Read the model definition and answer for the solid it produces. Units are mm, in the model's axes. Face numbers are marked on the shaded views. A direction names the side the tool comes from. Round coordinates to 2 decimals unless told otherwise and drop trailing zeros. Order: outer loops, then holes, each group sorted by start corner. A loop starts at its lowest first (then second) coordinate and runs counter-clockwise, first axis right, second up. Notation, with made-up numbers: (37, 44.5) - (46, 44.5) arc R21 ccw to (46, 83.5) - close; hole circle Ø4 at (-23.75, 34.25). An arc over 180 degrees is marked (long way). Answer as a JSON object with one key per item and string values. Group by question number.
Q1. A cutting plane is placed at D-D on x = 13. Determine the outline of the cut face in (y, z).
Q2. Consider line 1 (Z direction, x = 43, y = 2.5); line 2 (Z direction, x = 31.5, y = 14); line 3 (X direction, y = 8, z = 31.5). Determine where each line is inside the solid, lowest interval first.
Q3. A cutting plane is placed at A-A on z = 21. Determine the outline of the cut face in (x, y), and give its area (3 significant figures).
Q4. A cutting plane is placed at C-C on y = 16. Determine the outline of the cut face in (x, z).
Q5. The mould has two halves that part along X. Classify the marked faces 4, 5, 6 and 7: pulls with the +X half, pulls with the -X half, needs draft (parallel to the pull), parting line crosses it, or undercut.
Q6. Given pin 1 Ø2 at (y, z) = (5, 14) entering from -X; pin 2 Ø1.4 at (y, z) = (12.5, 40) entering from +X, each flat-ended and moving along its own axis, determine where each tip first touches the part or whether it passes through.
Q7. A tool of negligible diameter and unlimited length cuts with its end or side. For the marked faces 1, 2 and 3, from which of +Z, -Z, +X, -X, +Y, -Y can it reach the whole face along a straight path? Write none if from no direction.
Q8. A cutting plane is placed at B-B on x = 46. Determine the outline of the cut face in (y, z).
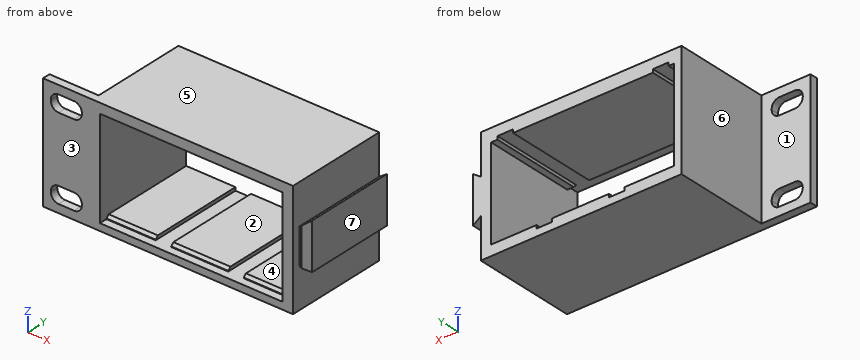
```python
from build123d import *

# Parameters (mm, degrees)
BOX027_W               = 71
BOX027_H               = 10
BOX027_DEPTH           = 10
BOX027_PLACEMENT_ANGLE = 45
BOX022_W               = 22
BOX022_H               = 37
BOX022_DEPTH           = 4
BOX023_W               = 18
BOX023_H               = 37
BOX023_DEPTH           = 4
BOX021_W               = 19
BOX021_H               = 37
BOX021_DEPTH           = 4
BOX028_W               = 80
BOX028_H               = 10
BOX028_DEPTH           = 10
BOX028_PLACEMENT_ANGLE = 315
BOX025_W               = 3
BOX025_H               = 37
BOX025_DEPTH           = 4
BOX026_W               = 4
BOX026_H               = 37
BOX026_DEPTH           = 4
BOX024_W               = 54
BOX024_H               = 37
BOX024_DEPTH           = 4
BOX019_W               = 12
BOX019_H               = 10
BOX019_DEPTH           = 6.3
FILLET_R               = 3
BOX020_W               = 12
BOX020_H               = 10
BOX020_DEPTH           = 6.3
FILLET001_R            = 3
BOX018_W               = 19
BOX018_H               = 37
BOX018_DEPTH           = 45
BOX017_W               = 70.5
BOX017_H               = 45
BOX017_DEPTH           = 37.95
BOX016_W               = 96.5
BOX016_H               = 40
BOX016_DEPTH           = 44.5
BOX013_W               = 3
BOX013_H               = 37
BOX013_DEPTH           = 17.92
BOX013_PLACEMENT_ANGLE = 45
BOX014_W               = 3
BOX014_H               = 37
BOX014_DEPTH           = 17.92
BOX014_PLACEMENT_ANGLE = 55
BOX015_W               = 3
BOX015_H               = 37
BOX015_DEPTH           = 17.92
BOX015_PLACEMENT_ANGLE = 125
BOX012_W               = 3
BOX012_H               = 37
BOX012_DEPTH           = 17.92
CUT007_PLACEMENT_ANGLE = 180


with BuildPart() as cube027:
    # Box027 → Box027 (new body)
    with BuildSketch(Plane.XY):
        with Locations((35.5, 5)):
            Rectangle(BOX027_W, BOX027_H)
    extrude(amount=BOX027_DEPTH)


with BuildPart() as cube027_1:
    # Box027 placement: moved
    add(cube027.part.moved(Location((22, -3, 0))).rotate(Axis((22, -3, 0), (1, 0, 0)), BOX027_PLACEMENT_ANGLE))


with BuildPart() as cube022:
    # Box022 → Box022 (new body)
    with BuildSketch(Plane(origin=(47, 0, 0), x_dir=(1, 0, 0), z_dir=(0, 0, 1))):
        with Locations((11, 18.5)):
            Rectangle(BOX022_W, BOX022_H)
    extrude(amount=BOX022_DEPTH)


with BuildPart() as cube023:
    # Box023 → Box023 (new body)
    with BuildSketch(Plane(origin=(75, 0, 0), x_dir=(1, 0, 0), z_dir=(0, 0, 1))):
        with Locations((9, 18.5)):
            Rectangle(BOX023_W, BOX023_H)
    extrude(amount=BOX023_DEPTH)


with BuildPart() as cut010:
    # Box021 → Box021 (new body)
    with BuildSketch(Plane(origin=(22, 0, 0), x_dir=(1, 0, 0), z_dir=(0, 0, 1))):
        with Locations((9.5, 18.5)):
            Rectangle(BOX021_W, BOX021_H)
    extrude(amount=BOX021_DEPTH)

    # Fusion005: union Cube022, Cube023
    add(cube022.part)
    add(cube023.part)

    # Cut010: cut Cube027
    add(cube027_1.part, mode=Mode.SUBTRACT)


with BuildPart() as cube028:
    # Box028 → Box028 (new body)
    with BuildSketch(Plane.XY):
        with Locations((40, 5)):
            Rectangle(BOX028_W, BOX028_H)
    extrude(amount=BOX028_DEPTH)


with BuildPart() as cube028_1:
    # Box028 placement: moved
    add(cube028.part.moved(Location((13, -8, 35))).rotate(Axis((13, -8, 35), (1, 0, 0)), BOX028_PLACEMENT_ANGLE))


with BuildPart() as cube025:
    # Box025 → Box025 (new body)
    with BuildSketch(Plane(origin=(21.05, 0, 39.45), x_dir=(1, 0, 0), z_dir=(0, 0, 1))):
        with Locations((1.5, 18.5)):
            Rectangle(BOX025_W, BOX025_H)
    extrude(amount=BOX025_DEPTH)


with BuildPart() as cube026:
    # Box026 → Box026 (new body)
    with BuildSketch(Plane(origin=(90.05, 0, 39.45), x_dir=(1, 0, 0), z_dir=(0, 0, 1))):
        with Locations((2, 18.5)):
            Rectangle(BOX026_W, BOX026_H)
    extrude(amount=BOX026_DEPTH)


with BuildPart() as cut011:
    # Box024 → Box024 (new body)
    with BuildSketch(Plane(origin=(30.05, 0, 39.45), x_dir=(1, 0, 0), z_dir=(0, 0, 1))):
        with Locations((27, 18.5)):
            Rectangle(BOX024_W, BOX024_H)
    extrude(amount=BOX024_DEPTH)

    # Fusion006: union Cube025, Cube026
    add(cube025.part)
    add(cube026.part)

    # Cut011: cut Cube028
    add(cube028_1.part, mode=Mode.SUBTRACT)


with BuildPart() as fillet_body:
    # Box019 → Box019 (new body)
    with BuildSketch(Plane(origin=(3, -3, 3.2), x_dir=(1, 0, 0), z_dir=(0, 0, 1))):
        with Locations((6, 5)):
            Rectangle(BOX019_W, BOX019_H)
    extrude(amount=BOX019_DEPTH)

    # Fillet
    fillet_edges = [fillet_body.edges().sort_by_distance(p)[0] for p in [
        (3, 2, 9.5),
        (3, 2, 3.2),
        (15, 2, 9.5),
        (15, 2, 3.2),
    ]]
    fillet(fillet_edges, radius=FILLET_R)


with BuildPart() as fillet_body_1:
    # Fillet placement: moved
    add(fillet_body.part.moved(Location((0, -1, 0))))


with BuildPart() as fillet001:
    # Box020 → Box020 (new body)
    with BuildSketch(Plane(origin=(3, -3, 3.2), x_dir=(1, 0, 0), z_dir=(0, 0, 1))):
        with Locations((6, 5)):
            Rectangle(BOX020_W, BOX020_H)
    extrude(amount=BOX020_DEPTH)

    # Fillet001
    fillet001_edges = [fillet001.edges().sort_by_distance(p)[0] for p in [
        (3, 2, 9.5),
        (3, 2, 3.2),
        (15, 2, 9.5),
        (15, 2, 3.2),
    ]]
    fillet(fillet001_edges, radius=FILLET001_R)


with BuildPart() as fillet001_1:
    # Fillet001 placement: moved
    add(fillet001.part.moved(Location((0, -1, 31.7))))


with BuildPart() as fusion004:
    # Box018 → Box018 (new body)
    with BuildSketch(Plane.XY):
        with Locations((9.5, 18.5)):
            Rectangle(BOX018_W, BOX018_H)
    extrude(amount=BOX018_DEPTH)

    # Fusion004: union Fillet body, Fillet001
    add(fillet_body_1.part)
    add(fillet001_1.part)


with BuildPart() as cube017:
    # Box017 → Box017 (new body)
    with BuildSketch(Plane(origin=(22, -4, 2.75), x_dir=(1, 0, 0), z_dir=(0, 0, 1))):
        with Locations((35.25, 22.5)):
            Rectangle(BOX017_W, BOX017_H)
    extrude(amount=BOX017_DEPTH)


with BuildPart() as cube016:
    # Box016 → Box016 (new body)
    with BuildSketch(Plane(origin=(0, -3, 0), x_dir=(1, 0, 0), z_dir=(0, 0, 1))):
        with Locations((48.25, 20)):
            Rectangle(BOX016_W, BOX016_H)
    extrude(amount=BOX016_DEPTH)


with BuildPart() as cube013:
    # Box013 → Box013 (new body)
    with BuildSketch(Plane.XY):
        with Locations((1.5, 18.5)):
            Rectangle(BOX013_W, BOX013_H)
    extrude(amount=BOX013_DEPTH)


with BuildPart() as cube013_1:
    # Box013 placement: moved
    add(cube013.part.moved(Location((314.75, -3, 13.25))).rotate(Axis((314.75, -3, 13.25), (0, 0, 1)), BOX013_PLACEMENT_ANGLE))


with BuildPart() as cube014:
    # Box014 → Box014 (new body)
    with BuildSketch(Plane.XY):
        with Locations((1.5, 18.5)):
            Rectangle(BOX014_W, BOX014_H)
    extrude(amount=BOX014_DEPTH)


with BuildPart() as cube014_1:
    # Box014 placement: moved
    add(cube014.part.moved(Location((313, 0, 12.75))).rotate(Axis((313, 0, 12.75), (0, 1, 0)), BOX014_PLACEMENT_ANGLE))


with BuildPart() as fusion002:
    # Box015 → Box015 (new body)
    with BuildSketch(Plane.XY):
        with Locations((1.5, 18.5)):
            Rectangle(BOX015_W, BOX015_H)
    extrude(amount=BOX015_DEPTH)


with BuildPart() as fusion002_1:
    # Box015 placement: moved
    add(fusion002.part.moved(Location((313, 0, 35.35))).rotate(Axis((313, 0, 35.35), (0, 1, 0)), BOX015_PLACEMENT_ANGLE))

    # Fusion002: union Cube014
    add(cube014_1.part)


with BuildPart() as rack_left_side_shorter:
    # Box012 → Box012 (new body)
    with BuildSketch(Plane(origin=(313.75, 0, 13.25), x_dir=(1, 0, 0), z_dir=(0, 0, 1))):
        with Locations((1.5, 18.5)):
            Rectangle(BOX012_W, BOX012_H)
    extrude(amount=BOX012_DEPTH)

    # Cut006: cut Fusion002
    add(fusion002_1.part, mode=Mode.SUBTRACT)

    # Cut007: cut Cube013
    add(cube013_1.part, mode=Mode.SUBTRACT)


with BuildPart() as rack_left_side_shorter_1:
    # Cut007 placement: moved
    add(rack_left_side_shorter.part.moved(Location((413.25, 0, 44.45))).rotate(Axis((413.25, 0, 44.45), (0, 1, 0)), CUT007_PLACEMENT_ANGLE))

    # Fusion003: union Cube016
    add(cube016.part)

    # Cut008: cut Cube017
    add(cube017.part, mode=Mode.SUBTRACT)

    # Cut009: cut Fusion004
    add(fusion004.part, mode=Mode.SUBTRACT)

    # Fusion007: union Cut010, Cut011
    add(cut010.part)
    add(cut011.part)


solid = rack_left_side_shorter_1.part
```
Result set:
{
 "1": {"outline": "(-3, 0) - (0, 0) - (0, 3.37) - (-3, 3.37) - close; (-3, 9.33) - (0, 9.33) - (0, 35.07) - (-3, 35.07) - close; (-3, 41.03) - (0, 41.03) - (0, 44.5) - (-3, 44.5) - close"},
 "2": {"line 1": "z = 0 to 2.75, 39.45 to 44.5", "line 2": "z = 0 to 4, 39.45 to 44.5", "line 3": "x = 19 to 22, 92.5 to 96.5"},
 "3": {"outline": "(0, -3) - (22, -3) - (22, 37) - (19, 37) - (19, 0) - (0, 0) - close; (92.5, -3) - (96.5, -3) - (96.5, 0) - (97.26, 0) - (99.5, 2.24) - (99.5, 37) - (92.5, 37) - close", "area": "445 mm²"},
 "4": {"outline": "(19, 0) - (96.5, 0) - (96.5, 15.39) - (99.5, 13.29) - (99.5, 31.17) - (96.5, 29.07) - (96.5, 44.5) - (19, 44.5) - close; hole (22, 4) - (41, 4) - (41, 2.75) - (47, 2.75) - (47, 4) - (69, 4) - (69, 2.75) - (75, 2.75) - (75, 4) - (92.5, 4) - (92.5, 39.45) - (90.05, 39.45) - (90.05, 40.7) - (84.05, 40.7) - (84.05, 39.45) - (30.05, 39.45) - (30.05, 40.7) - (24.05, 40.7) - (24.05, 39.45) - (22, 39.45) - close"},
 "5": {"face 4": "undercut", "face 5": "needs draft", "face 6": "pulls with the -X half", "face 7": "pulls with the +X half"},
 "6": {"pin 1": "stops at x = 19", "pin 2": "stops at x = 96.5"},
 "7": {"face 1": "+Z, -Z, -X, +Y", "face 2": "+Y, -Y", "face 3": "+Z, -Z, +X, -X, -Y"},
 "8": {"outline": "(-3, 0) - (37, 0) - (37, 2.75) - (-3, 2.75) - close; (-3, 40.7) - (0.44, 40.7) - (1.69, 39.45) - (37, 39.45) - (37, 44.5) - (-3, 44.5) - close"}
}
